```python
from build123d import *

# Parameters (mm, degrees)
SKETCH1_W           = 76.2
SKETCH1_H           = 38.1
SKETCH1_W_2         = 71.12
SKETCH1_H_2         = 33.02
EXTRUDE_THIN1_DEPTH = 261.62
CUT_EXTRUDE2_DEPTH  = 39.1
SKETCH4_R           = 19.05
CUT_EXTRUDE3_DEPTH  = 39.1
SKETCH5_R           = 1.3462
CUT_EXTRUDE6_DEPTH  = 77.2


with BuildPart() as part:
    # Sketch1 → Extrude-Thin1 (new body)
    with BuildSketch(Plane.XY):
        Rectangle(SKETCH1_W, SKETCH1_H)
        Rectangle(SKETCH1_W_2, SKETCH1_H_2, mode=Mode.SUBTRACT)
    extrude(amount=EXTRUDE_THIN1_DEPTH)

    # Sketch3 → Cut-Extrude2 (cut, through all)
    with BuildSketch(Plane(origin=(0, 19.05, 0), x_dir=(1, 0, 0), z_dir=(0, 1, 0))):
        with BuildLine():
            ThreePointArc((23.8125, -261.62), (21.931629786, -252.344291339), (16.586146516, -244.53389746))
            ThreePointArc((16.586146516, -244.53389746), (0, -237.8075), (-16.586146516, -244.53389746))
            ThreePointArc((-16.586146516, -244.53389746), (-21.931629786, -252.344291339), (-23.8125, -261.62))
            Line((-23.8125, -261.62), (23.8125, -261.62))
        make_face()
        with BuildLine():
            ThreePointArc((-23.8125, -261.62), (0, -285.4325), (23.8125, -261.62))
            Line((23.8125, -261.62), (-23.8125, -261.62))
        make_face()
        with BuildLine():
            Line((38.1, -261.62), (38.1, -244.53389746))
            Line((38.1, -244.53389746), (16.586146516, -244.53389746))
            ThreePointArc((16.586146516, -244.53389746), (21.931629786, -252.344291339), (23.8125, -261.62))
            Line((23.8125, -261.62), (38.1, -261.62))
        make_face()
        with BuildLine():
            ThreePointArc((-23.8125, -261.62), (-21.931629786, -252.344291339), (-16.586146516, -244.53389746))
            Line((-16.586146516, -244.53389746), (-38.1, -244.53389746))
            Line((-38.1, -244.53389746), (-38.1, -261.62))
            Line((-38.1, -261.62), (-23.8125, -261.62))
        make_face()
        with BuildLine():
            ThreePointArc((-16.586146516, -17.08610254), (0, -23.8125), (16.586146516, -17.08610254))
            ThreePointArc((16.586146516, -17.08610254), (21.931629786, -9.275708661), (23.8125, 0))
            Line((23.8125, 0), (-23.8125, 0))
            ThreePointArc((-23.8125, 0), (-21.931629786, -9.275708661), (-16.586146516, -17.08610254))
        make_face()
        with BuildLine():
            Line((-23.8125, 0), (23.8125, 0))
            ThreePointArc((23.8125, 0), (0, 23.8125), (-23.8125, 0))
        make_face()
        with BuildLine():
            Line((-38.1, -17.08610254), (-16.586146516, -17.08610254))
            ThreePointArc((-16.586146516, -17.08610254), (-21.931629786, -9.275708661), (-23.8125, 0))
            Line((-23.8125, 0), (-38.1, 0))
            Line((-38.1, 0), (-38.1, -17.08610254))
        make_face()
        with BuildLine():
            Line((16.586146516, -17.08610254), (38.1, -17.08610254))
            Line((38.1, -17.08610254), (38.1, 0))
            Line((38.1, 0), (23.8125, 0))
            ThreePointArc((23.8125, 0), (21.931629786, -9.275708661), (16.586146516, -17.08610254))
        make_face()
    extrude(amount=-CUT_EXTRUDE2_DEPTH, mode=Mode.SUBTRACT)

    # Sketch4 → Cut-Extrude3 (cut, through all)
    with BuildSketch(Plane(origin=(0, 19.05, 0), x_dir=(1, 0, 0), z_dir=(0, 1, 0))):
        with Locations((0, -179.44639746)):
            Circle(SKETCH4_R)
        with Locations((0, -82.17360254)):
            Circle(SKETCH4_R)
    extrude(amount=-CUT_EXTRUDE3_DEPTH, mode=Mode.SUBTRACT)

    # Sketch5 → Cut-Extrude6 (cut, through all)
    with BuildSketch(Plane(origin=(38.1, 0, 0), x_dir=(0, 0, -1), z_dir=(1, 0, 0))):
        with Locations((-44.044847153, 0)):
            Circle(SKETCH5_R)
    extrude(amount=-CUT_EXTRUDE6_DEPTH, mode=Mode.SUBTRACT)


solid = part.part
```
Part model, mm, in its own coordinate system. A direction names the side the tool comes from. Give positions to 0.01 mm unless a question says otherwise; leave off trailing zeros. Order: outer loops, then holes, each group sorted by start corner. A loop starts at its lowest first (then second) coordinate and runs counter-clockwise, first axis right, second up. Notation, with made-up numbers: M 88,77 L 140,77 A29 ccw 140,107 Z; hole C 52.5,34.25 d11. An arc over 180 degrees is marked long. Use a Markdown table: item, result. Add a question column.
(1) Saw through at C-C, the plane x = 26.5. Give the cut face in (y, z), and give its area (3 significant figures).
(2) Drop flat-ended pins along their axis: P1, Ø8, axis at x = 3.5, y = 13.5, coming from the +Z side; P2, Ø3.5, axis at y = 0, z = 44.04, coming from the -X side; P3, Ø1.6, axis at y = 0, z = 44.04, coming from the -X side. Give the stop position or say it passes through.
(3) Mould opens along Y. For faces 3 (the face through (0, -16.51, 129)), 4 (the face through (-2.48, 17.798, 63.286)), 5 (the face through (-1, -19.05, 129)) say: +Y half, -Y half, draft (parallel to the pull), parting line (faces both ways), or undercut.
(4) Saw through at D-D, the plane z = 157. Give the cut face in (x, y).
(5) Saw through at B-B, the plane y = 5. Give the cut face in (x, z).
(6) Probe line 1 along Y through (x, z) = (-8, 61); line 2 along X through (y, z) = (-0.5, 233). List the from-to ranges inside material, lowest first. Write a range as [from, to].
(7) Saw through at A-A, the plane x = 0. Give the cut face in (y, z), and give its area (3 significant figures).
(8) 3-axis set-ups, long thin cutter, end or side, ignore diameter. For faces 1 (the face through (-35.56, 0, 129)), 2 (the face through (0.26, 17.8, 237.81)): which of +Z, -Z, +X, -X, +Y, -Y reach the whole face in a straight line?
Answer key:
| question | item | result |
|---|---|---|
| 1 | outline | M -19.05,17.09 L -16.51,17.09 L -16.51,244.53 L -19.05,244.53 Z; M 16.51,17.09 L 19.05,17.09 L 19.05,244.53 L 16.51,244.53 Z |
| 1 | area | 1,160 mm^2 |
| 2 | P1 | z = 238.61 |
| 2 | P2 | x = -38.1 |
| 2 | P3 | through |
| 3 | face 3 | undercut |
| 3 | face 4 | draft |
| 3 | face 5 | -Y half |
| 4 | outline | M -38.1,-19.05 L 38.1,-19.05 L 38.1,19.05 L -38.1,19.05 Z; hole M -35.56,-16.51 L 35.56,-16.51 L 35.56,16.51 L -35.56,16.51 Z |
| 5 | outline | M -38.1,17.09 L -35.56,17.09 L -35.56,244.53 L -38.1,244.53 Z; M 35.56,17.09 L 38.1,17.09 L 38.1,244.53 L 35.56,244.53 Z |
| 6 | line 1 | [-19.05, -16.51], [16.51, 19.05] |
| 6 | line 2 | [-38.1, -35.56], [35.56, 38.1] |
| 7 | outline | M -19.05,23.81 L -16.51,23.81 L -16.51,63.12 L -19.05,63.12 Z; M -19.05,101.22 L -16.51,101.22 L -16.51,160.4 L -19.05,160.4 Z; M -19.05,198.5 L -16.51,198.5 L -16.51,237.81 L -19.05,237.81 Z; M 16.51,23.81 L 19.05,23.81 L 19.05,63.12 L 16.51,63.12 Z; M 16.51,101.22 L 19.05,101.22 L 19.05,160.4 L 16.51,160.4 Z; M 16.51,198.5 L 19.05,198.5 L 19.05,237.81 L 16.51,237.81 Z |
| 7 | area | 700 mm^2 |
| 8 | face 1 | +Z, -Z |
| 8 | face 2 | +Z, +Y, -Y |
